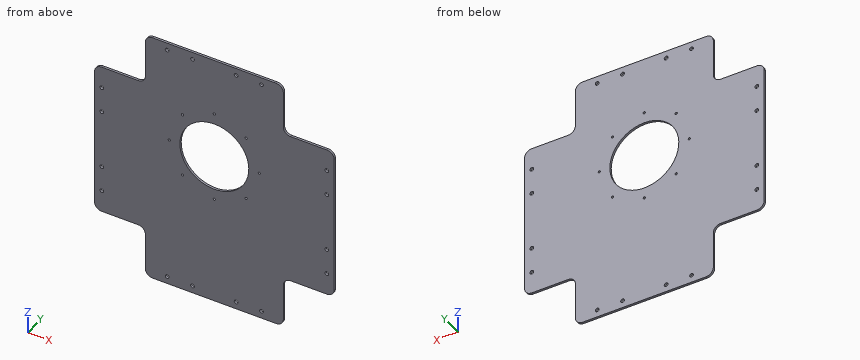
```python
from build123d import *

# Parameters (mm, degrees)
SKETCH1_R           = 56
BOSS_EXTRUDE1_DEPTH = 3
FILLET1_R           = 10
SKETCH2_R           = 2.6
SKETCH2_R_2         = 1.6
CUT_EXTRUDE1_DEPTH  = 482.049893462
BOSS_EXTRUDE2_START = -3
SKETCH3_R           = 56
SKETCH3_R_2         = 47.5
BOSS_EXTRUDE2_DEPTH = 3


with BuildPart() as part:
    # Sketch1 → Boss-Extrude1 (new body)
    with BuildSketch(Plane(origin=(0, 0, 0), x_dir=(1, 0, 0), z_dir=(0, 1, 0))):
        Polygon((70, 70), (70, 0), (260, 0), (260, 70), (330, 70), (330, 280), (260, 280), (260, 350), (70, 350), (70, 280), (0, 280), (0, 70), align=None)
        with Locations(Location((165, 140, 0), (0, 0, 270))):
            Circle(SKETCH1_R, mode=Mode.SUBTRACT)
    extrude(amount=BOSS_EXTRUDE1_DEPTH)

    # Fillet1
    fillet1_edges = [part.edges().sort_by_distance(p)[0] for p in [
        (70, 1.5, 0),
        (70, 1.5, -70),
        (0, 1.5, -70),
        (0, 1.5, -280),
        (70, 1.5, -280),
        (70, 1.5, -350),
        (260, 1.5, -350),
        (260, 1.5, -280),
        (330, 1.5, -280),
        (330, 1.5, -70),
        (260, 1.5, -70),
        (260, 1.5, 0),
    ]]
    fillet(fillet1_edges, radius=FILLET1_R)

    # Sketch2 → Cut-Extrude1 (cut, through all)
    with BuildSketch(Plane(origin=(0, 3, 0), x_dir=(1, 0, 0), z_dir=(0, 1, 0))):
        with Locations(Location((100, 340, 0), (0, 0, 270))):
            Circle(SKETCH2_R)
        with Locations(Location((135, 340, 0), (0, 0, 270))):
            Circle(SKETCH2_R)
        with Locations(Location((195, 340, 0), (0, 0, 270))):
            Circle(SKETCH2_R)
        with Locations(Location((230, 340, 0), (0, 0, 270))):
            Circle(SKETCH2_R)
        with Locations(Location((10, 250, 0), (0, 0, 270))):
            Circle(SKETCH2_R)
        with Locations(Location((10, 215, 0), (0, 0, 270))):
            Circle(SKETCH2_R)
        with Locations(Location((10, 100, 0), (0, 0, 270))):
            Circle(SKETCH2_R)
        with Locations(Location((10, 135, 0), (0, 0, 270))):
            Circle(SKETCH2_R)
        with Locations(Location((100, 10, 0), (0, 0, 270))):
            Circle(SKETCH2_R)
        with Locations(Location((135, 10, 0), (0, 0, 270))):
            Circle(SKETCH2_R)
        with Locations(Location((195, 10, 0), (0, 0, 270))):
            Circle(SKETCH2_R)
        with Locations(Location((230, 10, 0), (0, 0, 270))):
            Circle(SKETCH2_R)
        with Locations(Location((320, 100, 0), (0, 0, 270))):
            Circle(SKETCH2_R)
        with Locations(Location((320, 135, 0), (0, 0, 270))):
            Circle(SKETCH2_R)
        with Locations(Location((320, 250, 0), (0, 0, 270))):
            Circle(SKETCH2_R)
        with Locations(Location((320, 215, 0), (0, 0, 270))):
            Circle(SKETCH2_R)
        with Locations(Location((165, 202, 0), (0, 0, 270))):
            Circle(SKETCH2_R_2)
        with Locations(Location((208.840620434, 183.840620434, 0), (0, 0, 270))):
            Circle(SKETCH2_R_2)
        with Locations(Location((227, 140, 0), (0, 0, 270))):
            Circle(SKETCH2_R_2)
        with Locations(Location((208.840620434, 96.159379566, 0), (0, 0, 270))):
            Circle(SKETCH2_R_2)
        with Locations(Location((165, 78, 0), (0, 0, 270))):
            Circle(SKETCH2_R_2)
        with Locations(Location((121.159379566, 96.159379566, 0), (0, 0, 270))):
            Circle(SKETCH2_R_2)
        with Locations(Location((103, 140, 0), (0, 0, 270))):
            Circle(SKETCH2_R_2)
        with Locations(Location((121.159379566, 183.840620434, 0), (0, 0, 270))):
            Circle(SKETCH2_R_2)
    extrude(amount=-CUT_EXTRUDE1_DEPTH, mode=Mode.SUBTRACT)

    # Sketch3 → Boss-Extrude2 (add)
    with BuildSketch(Plane(origin=(0, 3, 0), x_dir=(1, 0, 0), z_dir=(0, 1, 0)).offset(BOSS_EXTRUDE2_START)):
        with Locations((165, 140)):
            Circle(SKETCH3_R)
        with Locations(Location((165, 140, 0), (0, 0, 270))):
            Circle(SKETCH3_R_2, mode=Mode.SUBTRACT)
    extrude(amount=BOSS_EXTRUDE2_DEPTH)


solid = part.part
```
Geometry: final body of the model. Coordinates: model frame, mm. Coordinates: 2 decimals unless noted, no trailing zeros. Write each loop counter-clockwise with the first axis right and the second up, starting at its lowest first coordinate (ties: lowest second). Pieces come first, ordered by that corner, then holes. Notation, with made-up numbers: M 73.5,30.25 L 92.5,30.25 A20 cw 92.5,63.25 Z; hole C 25.25,1.5 d6. An arc over 180 degrees is marked long. Answer as CSV lines item,"result". Start each with the question number.
Q1. Cut plane B-B on x = 34.5. Return the cut outline in (y, z), then the cut area to 3 significant figures.
Q2. Cut plane A-A on z = -171. Return the cut outline in (x, y).
Q3. Pin query (flat end, axial travel): P1, Ø4, axis at x = 320, z = -135, coming from the -Y side; P2, Ø1.5, axis at y = 2, z = -40.5, coming from the +X side; P3, Ø1.5, axis at x = 40.5, y = 1.5, coming from the -Z side. Return the tip coordinate at first contact, or that it passes through.
Q4. Line query: line 1 (X direction, y = 1.2, z = -250); line 2 (Z direction, x = 320, y = 1.7); line 3 (Z direction, x = 230, y = 1.6). Output: solid intervals per line, ascending. Write a range as from..to.
Q5. Cut plane D-D on y = 1.85. Count the separate pieces of the cut face and the enclosed holes in it, then the cut area to 3 significant figures.
Q6. Cut plane C-C on z = -43.5. Return the cut outline in (x, y), then the cut area to 3 significant figures.
Findings below:
1,outline,"M 0,-280 L 3,-280 L 3,-70 L 0,-70 Z"
1,area,"630 mm2"
2,outline,"M 0,0 L 129.01,0 L 129.01,3 L 0,3 Z; M 200.99,0 L 330,0 L 330,3 L 200.99,3 Z"
3,P1,"passes through"
3,P2,"stops at x = 260"
3,P3,"stops at z = -280"
4,line 1,"x = 0..7.4, 12.6..317.4, 322.6..330"
4,line 2,"z = -280..-252.6, -247.4..-217.6, -212.4..-137.6, -132.4..-102.6, -97.4..-70"
4,line 3,"z = -350..-342.6, -337.4..-12.6, -7.4..0"
5,separate pieces,"1"
5,enclosed holes,"25"
5,area,"88,300 mm2"
6,outline,"M 70,0 L 260,0 L 260,3 L 70,3 Z"
6,area,"570 mm2"
